```python
from build123d import *

# Parameters (mm, degrees)
FILLET1_R = 3
FILLET2_R = 1


with BuildPart() as part:
    # Sketch1 → Revolve1 (revolve)
    with BuildSketch(Plane.XY, mode=Mode.PRIVATE) as revolve1_sk:
        Polygon((0, 0), (0, 25), (3, 25), (3, 18), (2, 18), (2, 7), (3, 7), (3, 3), (4, 3), (4, 0), align=None)
    revolve(revolve1_sk.sketch.rotate(Axis((0, 0, 0), (0, 1, 0)), 90), axis=Axis((0, 0, 0), (0, 1, 0)))

    # Fillet1
    fillet1_edges = [part.edges().sort_by_distance(p)[0] for p in [
        (0, 25, 3),
    ]]
    fillet(fillet1_edges, radius=FILLET1_R)

    # Fillet2
    fillet2_edges = [part.edges().sort_by_distance(p)[0] for p in [
        (0, 18, 2),
        (0, 7, 2),
    ]]
    fillet(fillet2_edges, radius=FILLET2_R - 0.0001)  # a hair under: the kernel refuses the full size

    # Sketch2 → Cut-Revolve1 (revolve, cut)
    with BuildSketch(Plane.XY, mode=Mode.PRIVATE) as cut_revolve1_sk:
        with BuildLine():
            Line((0, 2.825522326), (0, 0))
            Line((0, 0), (2.825522326, 0))
            ThreePointArc((2.825522326, 0), (1.997945997, 1.997945997), (0, 2.825522326))
        make_face()
    revolve(cut_revolve1_sk.sketch.rotate(Axis((0, 2.825522326, 0), (0, -1, 0)), 270), axis=Axis((0, 2.825522326, 0), (0, -1, 0)), mode=Mode.SUBTRACT)


solid = part.part
```
Can you work these out from the model? Positions are in its coordinate system, mm. A direction names the side the tool comes from. Coordinates: 2 decimals unless noted, no trailing zeros. Order: outer loops, then holes, each group sorted by start corner. A loop starts at its lowest first (then second) coordinate and runs counter-clockwise, first axis right, second up.
1. Thinking about a two-plate mould opening in Y: for faces 3 (the face through (2, 12, 0)), 4 (the face through (-3, 3, 1)), 5 (the face through (-0.9, 4.97, -2.86)), which applies, +Y half, -Y half, draft (parallel to the pull), parting line (faces both ways), or undercut?
2. I'm going to push flat-ended pins straight in: pin 1 (3 mm diameter, centred on y = 20.5, z = 2.5, fed in from -X); pin 2 (2 mm diameter, centred on x = 0.5, y = 20, fed in from -Z); pin 3 (4 mm diameter, centred on y = 18.5, z = -1.5, fed in from +X). Where does each tip first touch, or does it pass through?
3. I need wall thicknesses on line 1 (Y direction, x = -2.5, z = 1.75); line 2 (Y direction, x = 2, z = -1.25); line 3 (Y direction, x = -1.75, z = 1.25). Which ranges of each line are inside material? Lowest first, please.
4. For faces 1 (the face through (-0.9, 19.97, -2.86)), 2 (the face through (1, 0, 3)), which set-ups out of +Z, -Z, +X, -X, +Y, -Y let a thin tool reach every point of the face, with its end or its side?
5. If we section it at D-D (y = 7.5): Please give me the cut outline in (x, z), then the cut area to 3 significant figures.
6. If we section it at C-C (y = 4): Please give me the cut outline in (x, z).
Entries:
1. face 3: undercut
1. face 4: +Y half
1. face 5: draft
2. pin 1: stops at x = -2.83
2. pin 2: stops at z = -3
2. pin 3: stops at x = 3
3. line 1: y = 0 to 3
3. line 2: y = 1.56 to 7.23, 17.77 to 23.85
3. line 3: y = 1.83 to 7.47, 17.53 to 24.09
4. face 1: +Y
4. face 2: +Z, -Z, +X, -X, -Y
5. outline: circle Ø4.27 at (0, 0)
5. area: 14.3 mm2
6. outline: circle Ø6 at (0, 0)
